Check sheet for the modelled part. Datum: model origin and axes. Units: mm. A direction names the side the tool comes from. Round coordinates to 2 decimals unless told otherwise and drop trailing zeros. Loops run counter-clockwise (first coordinate to the right, second up) from the corner with the lowest first, then second, coordinate; pieces in that order, holes last. Notation, with made-up numbers: (20.25, 70) -> (46.25, 70) arc R13 cw to (46.25, 79) -> close; hole circle Ø9 at (48.25, -3). An arc over 180 degrees is marked (long way). Use one line per item in the form item = value. Start each with the question number.
(1) Set-up check for faces 4 (the flat face through (0, 68.2, -7)), 5 (the flat face through (-15, 36.7, 0)), 6 (the cylindrical face through (-16.108, 11.191, -3.577)): record each of +Z, -Z, +X, -X, +Y, -Y from which the full face is reachable in a straight line by a thin tool's end or side.
(2) Sectioned sample at C-C (y = 14). Record the cut outline in (x, z).
(3) Draft check along Z on faces 1 (the flat face through (0, 46.7, 0)), 2 (the flat face through (8, 36.7, 13)), 3 (the cylindrical face through (4.88, -0.74, -1.08)). Enter one of: released by +Z, released by -Z, zero draft, split by the parting line, or undercut.
(4) Sectioned sample at A-A (z = 0). Record the cut outline in (x, y), and give its area (3 significant figures).
(5) Material ranges on probe 1 along X at (y, z) = (43, 0); probe 2 along Y at (x, z) = (2.5, 12.5); probe 3 along Y at (x, z) = (17, -6.5), recorded low to high. Write a range as [from, to].
(6) Sectioned sample at D-D (x = 0). Record the cut outline in (y, z).
(7) Go/stop test with flat-tipped pins: pin 1 (2.5 mm diameter, centred on x = 15, z = 0, fed in from +Y); pin 2 (1 mm diameter, centred on x = 5, y = 6.5, fed in from +Z); pin 3 (5 mm diameter, centred on y = 21.5, z = -13.5, fed in from +X). Record where each tip stops, or that it passes through.
(8) Sectioned sample at B-B (x = 15.5). Record the cut outline in (y, z).
from build123d import *

# Parameters (mm, degrees)
SKETCH_1_R          = 16.5
EXTRUDE_1_DEPTH     = 22.7
SKETCH_2_R          = 18.5
EXTRUDE_2_DEPTH     = 24
SKETCH_3_R          = 6
EXTRUDE_3_DEPTH     = 6
SKETCH_4_R          = 3
EXTRUDE_4_DEPTH     = 15.5
CUT_EXTRUDE_1_DEPTH = 12
SKETCH_6_R          = 1.5
CUT_EXTRUDE_2_DEPTH = 10
SKETCH_7_R          = 5
EXTRUDE_5_DEPTH     = 2
FILLET_1_R          = 0.5


with BuildPart() as part:
    # 草图1 → 凸台-拉伸1 (new body)
    with BuildSketch(Plane(origin=(0, 0, 0), x_dir=(1, 0, 0), z_dir=(0, 1, 0))):
        with Locations(Location((0, 0, 0), (0, 0, 270))):
            Circle(SKETCH_1_R)
    extrude(amount=EXTRUDE_1_DEPTH)

    # 草图2 → 凸台-拉伸2 (add)
    with BuildSketch(Plane(origin=(0, 22.7, 0), x_dir=(1, 0, 0), z_dir=(0, 1, 0))):
        with Locations(Location((0, 0, 0), (0, 0, 270))):
            Circle(SKETCH_2_R)
    extrude(amount=EXTRUDE_2_DEPTH)

    # 草图3 → 凸台-拉伸3 (add)
    with BuildSketch(Plane(origin=(0, 46.7, 0), x_dir=(1, 0, 0), z_dir=(0, 1, 0))):
        with Locations(Location((0, 7, 0), (0, 0, 270))):
            Circle(SKETCH_3_R)
    extrude(amount=EXTRUDE_3_DEPTH)

    # 草图4 → 凸台-拉伸4 (add)
    with BuildSketch(Plane(origin=(0, 52.7, 0), x_dir=(1, 0, 0), z_dir=(0, 1, 0))):
        with Locations(Location((0, 7, 0), (0, 0, 270))):
            Circle(SKETCH_4_R)
    extrude(amount=EXTRUDE_4_DEPTH)

    # 草图5 → 切除-拉伸1 (cut)
    with BuildSketch(Plane(origin=(0, 68.2, 0), x_dir=(1, 0, 0), z_dir=(0, 1, 0))):
        Polygon((-80.661429966, 9.5), (-1.658312395, 9.5), (1.658312395, 9.5), (80.661429966, 9.5), (80.661429966, 167.506235142), (-80.661429966, 167.506235142), align=None)
    extrude(amount=-CUT_EXTRUDE_1_DEPTH, mode=Mode.SUBTRACT)

    # 草图6 → 切除-拉伸2 (cut)
    with BuildSketch(Plane(origin=(0, 46.7, 0), x_dir=(1, 0, 0), z_dir=(0, 1, 0))):
        with Locations(Location((15.5, 0, 0), (0, 0, 270))):
            Circle(SKETCH_6_R)
        with Locations(Location((7.75, -13.423393759, 0), (0, 0, 270))):
            Circle(SKETCH_6_R)
        with Locations(Location((-7.75, -13.423393759, 0), (0, 0, 270))):
            Circle(SKETCH_6_R)
        with Locations(Location((-15.5, 0, 0), (0, 0, 270))):
            Circle(SKETCH_6_R)
        with Locations(Location((-7.75, 13.423393759, 0), (0, 0, 270))):
            Circle(SKETCH_6_R)
        with Locations(Location((7.75, 13.423393759, 0), (0, 0, 270))):
            Circle(SKETCH_6_R)
    extrude(amount=-CUT_EXTRUDE_2_DEPTH, mode=Mode.SUBTRACT)

    # 草图7 → 凸台-拉伸5 (add)
    with BuildSketch(Plane.XZ):
        with Locations(Location((0, 0, 0), (0, 0, 90))):
            Circle(SKETCH_7_R)
    extrude(amount=EXTRUDE_5_DEPTH)

    # 圆角1
    fillet_1_edges = [part.edges().sort_by_distance(p)[0] for p in [
        (0, -2, -5),
    ]]
    fillet(fillet_1_edges, radius=FILLET_1_R)


solid = part.part
Checks:
q1.face_4 = +Z, -Z, +X, -X, +Y
q1.face_5 = +Y
q1.face_6 = -Y
q2.outline = circle Ø33 at (0, 0)
q3.face_1 = zero draft
q3.face_2 = undercut
q3.face_3 = split by the parting line
q4.outline = (-18.5, 22.7) -> (-16.5, 22.7) -> (-16.5, 0) -> (-5, 0) -> (-5, -1.5) arc R0.5 ccw to (-4.5, -2) -> (4.5, -2) arc R0.5 ccw to (5, -1.5) -> (5, 0) -> (16.5, 0) -> (16.5, 22.7) -> (18.5, 22.7) -> (18.5, 46.7) -> (17, 46.7) -> (17, 36.7) -> (14, 36.7) -> (14, 46.7) -> (-14, 46.7) -> (-14, 36.7) -> (-17, 36.7) -> (-17, 46.7) -> (-18.5, 46.7) -> close
q4.area = 1,600 mm2
q5.probe_1 = [-18.5, -17], [-14, 14], [17, 18.5]
q5.probe_2 = [0, 46.7]
q5.probe_3 = [22.7, 46.7]
q6.outline = (-2, -4.5) arc R0.5 ccw to (-1.5, -5) -> (0, -5) -> (0, -16.5) -> (22.7, -16.5) -> (22.7, -18.5) -> (46.7, -18.5) -> (46.7, -13) -> (52.7, -13) -> (52.7, -10) -> (56.2, -10) -> (56.2, -9.5) -> (68.2, -9.5) -> (68.2, -4) -> (52.7, -4) -> (52.7, -1) -> (46.7, -1) -> (46.7, 18.5) -> (22.7, 18.5) -> (22.7, 16.5) -> (0, 16.5) -> (0, 5) -> (-1.5, 5) arc R0.5 ccw to (-2, 4.5) -> close
q7.pin_1 = 46.7
q7.pin_2 = 15.87
q7.pin_3 = 14.64
q8.outline = (0, -5.66) -> (22.7, -5.66) -> (22.7, -10.1) -> (46.7, -10.1) -> (46.7, -1.5) -> (36.7, -1.5) -> (36.7, 1.5) -> (46.7, 1.5) -> (46.7, 10.1) -> (22.7, 10.1) -> (22.7, 5.66) -> (0, 5.66) -> close
